Here's the drawing with two shaded views (mm, measured from the low corner). I have some questions. A direction names the side the tool comes from. Give positions to 0.01 mm unless a question says otherwise; leave off trailing zeros. Order: outer loops, then holes, each group sorted by start corner. A loop starts at its lowest first (then second) coordinate and runs counter-clockwise, first axis right, second up. Notation, with made-up numbers: M -20,-10.75 L 34,-10.75 A22 cw 34,-0.75 Z; hole C -18,6.25 d4. An arc over 180 degrees is marked long. Use a Markdown table: item, result. Add a question column.
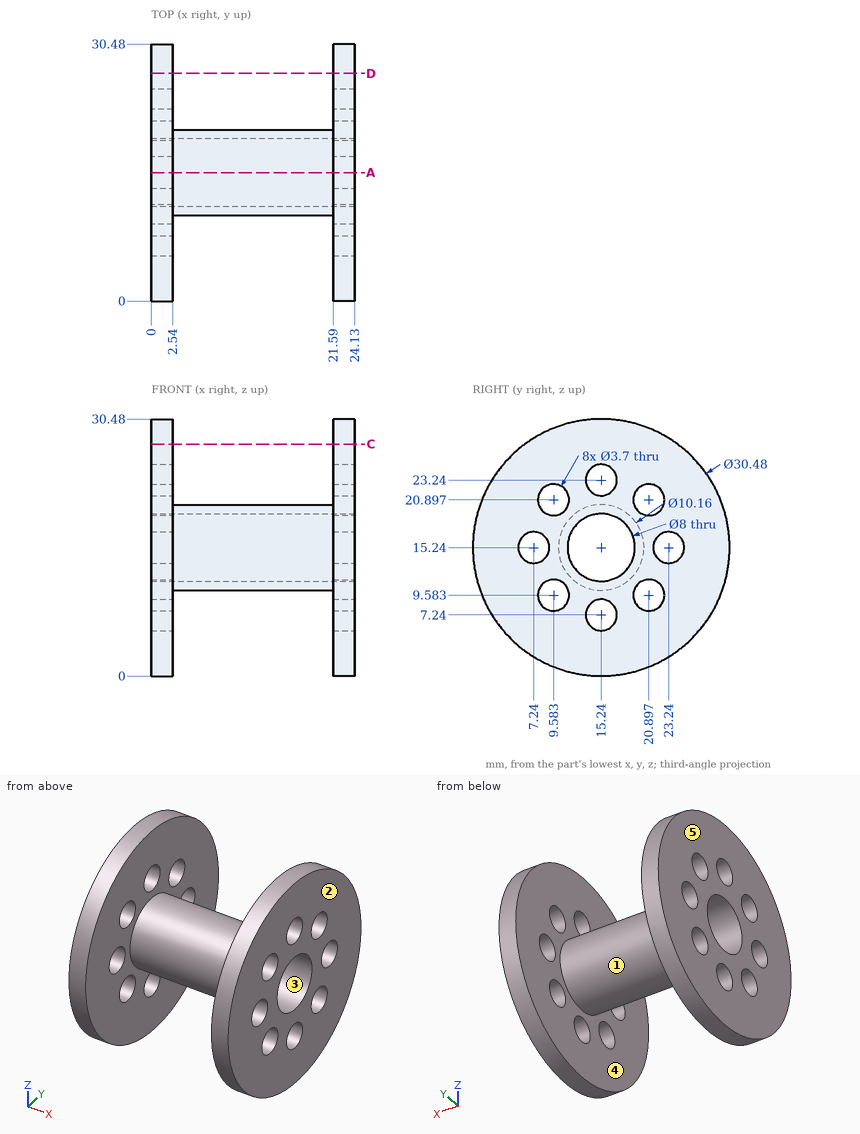
1) Suppose I cut it at A-A on y = 15.24. Count the separate pieces of the cut face and the enclosed holes in it, and give its area (3 significant figures).
2) We'd pull the mould along Y, two halves only. Please class the marked faces 1, 2 and 3: pulls with the +Y half, pulls with the -Y half, needs draft (parallel to the pull), parting line crosses it, or undercut.
3) For pin 1 (6 mm diameter, centred on x = 6, z = 21, fed in from -Y) (1 decimal); pin 2 (5 mm diameter, centred on x = 20.5, z = 10.5, fed in from -Y) (3 decimals); pin 3 (3 mm diameter, centred on x = 2.5, y = 22.5, fed in from -Z), each with a flat end and sliding along its axis, tell me the tip position at first contact or that it passes through.
4) Please list where these lines run through material, in increasing order: line 1 (X direction, y = 24, z = 3); line 2 (Y direction, x = 19, z = 18) (1 decimal); line 3 (Z direction, x = 22.75, y = 28). Write a range as from..to.
5) Suppose I cut it at D-D on y = 27. Please give me the cut outline in (x, z).
6) For the marked faces 4 and 5, which set-ups out of +Z, -Z, +X, -X, +Y, -Y let a thin tool reach every point of the face, with its end or its side?
7) Suppose I cut it at C-C on z = 27.5. Please give me the cut outline in (x, y).
Values found:
| question | item | result |
|---|---|---|
| 1 | separate pieces | 6 |
| 1 | enclosed holes | 0 |
| 1 | area | 118 mm^2 |
| 2 | face 1 | parting line crosses it |
| 2 | face 2 | needs draft |
| 2 | face 3 | undercut |
| 3 | pin 1 | stops at y = 11 |
| 3 | pin 2 | stops at y = 0.205 |
| 3 | pin 3 | stops at z = 1.13 |
| 4 | line 1 | x = 0..2.54, 21.59..24.13 |
| 4 | line 2 | y = 11..12.3, 18.1..19.5 |
| 4 | line 3 | z = 6.91..23.57 |
| 5 | outline | M 0,5.55 L 2.54,5.55 L 2.54,24.93 L 0,24.93 Z; M 21.59,5.55 L 24.13,5.55 L 24.13,24.93 L 21.59,24.93 Z |
| 6 | face 4 | none |
| 6 | face 5 | +Z, -Z, -X, +Y, -Y |
| 7 | outline | M 0,6.19 L 2.54,6.19 L 2.54,24.29 L 0,24.29 Z; M 21.59,6.19 L 24.13,6.19 L 24.13,24.29 L 21.59,24.29 Z |
